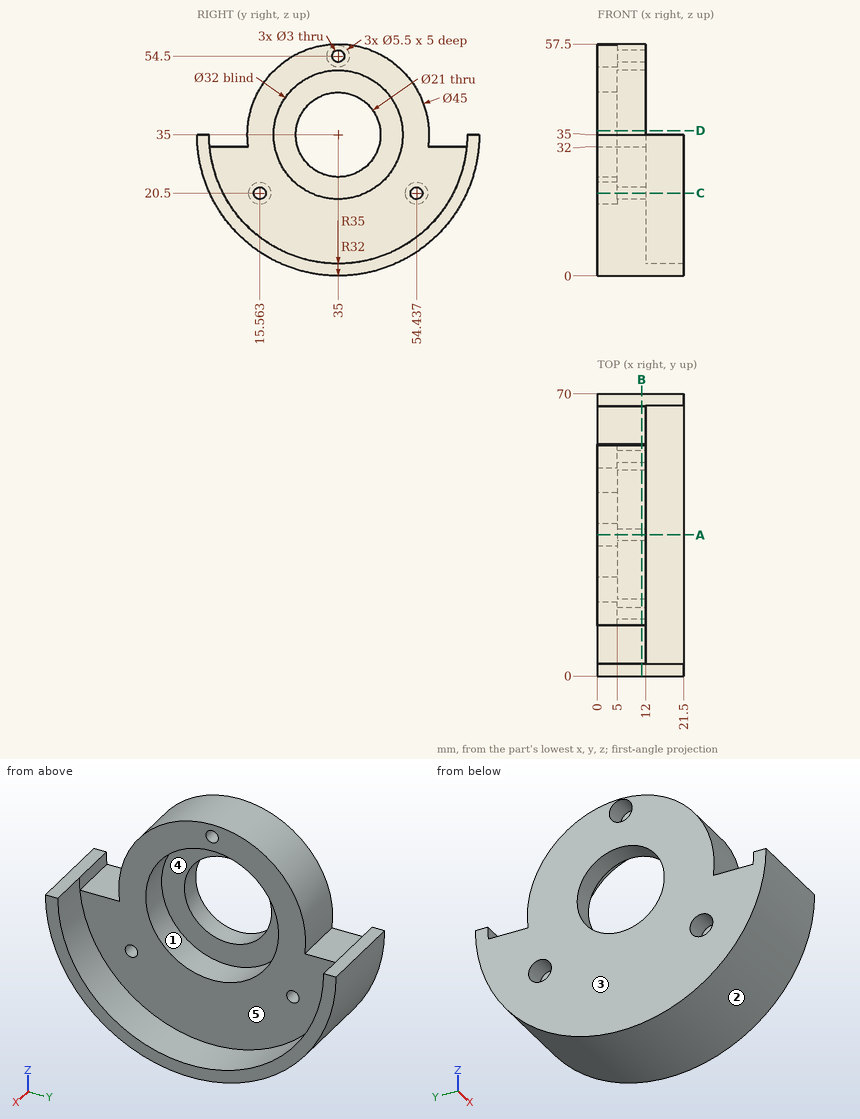
Geometry: see drawing. Coordinates: mm, zero at the bounding-box minimum. A direction names the side the tool comes from. Give positions to 0.01 mm unless a question says otherwise; leave off trailing zeros. Loops run counter-clockwise (first coordinate to the right, second up) from the corner with the lowest first, then second, coordinate; pieces in that order, holes last. Notation, with made-up numbers: (78, 14) - (101, 14) arc R14 cw to (101, 40) - close; hole circle Ø5 at (85, -30.75). An arc over 180 degrees is marked (long way). Use CSV: the item, a comma, the result in double quotes. Start each with the question number.
Item 1: Section C-C on z = 20.5. Return loops of the section in (x, y) (1 decimal).
Item 2: Section D-D on z = 36. Return loops of the section in (x, y).
Item 3: Mould query, pull axis Z, two halves, no side actions, for the marked faces 1, 2 and 3. Classes: pulls with the +Z half, pulls with the -Z half, needs draft (parallel to the pull), parting line crosses it, or undercut.
Item 4: Contact query for flat-ended pins moving along their axis: P1, Ø3, axis at y = 32, z = 41.5, coming from the -X side; P2, Ø10.5, axis at x = 5, y = 63.5, coming from the +Z side; P3, Ø8, axis at x = 12.5, z = 8, coming from the -Y side; P4, Ø4, axis at x = 11.5, z = 24, coming from the -Y side. Output: stop coordinate, or through.
Item 5: Section B-B on x = 11. Return loops of the section in (y, z).
Item 6: Line query: line 1 (Z direction, x = 8.75, y = 34.5) (1 decimal); line 2 (Y direction, x = 7.25, z = 20.5) (1 decimal); line 3 (X direction, y = 49, z = 15). Output: solid intervals per line, ascending.
Item 7: Reachability of the marked faces 4 and 5 from +Z, -Z, +X, -X, +Y, -Y: full face, straight path, thin tool, end or side. Return the list, or none.
Item 8: Section A-A on y = 35. Return loops of the section in (x, z).
Ans:
1,outline,"(0, 3.1) - (21.5, 3.1) - (21.5, 6.5) - (12, 6.5) - (12, 14.1) - (5, 14.1) - (5, 12.8) - (0, 12.8) - close; (0, 18.3) - (5, 18.3) - (5, 17.1) - (12, 17.1) - (12, 28.2) - (5, 28.2) - (5, 41.8) - (12, 41.8) - (12, 52.9) - (5, 52.9) - (5, 51.7) - (0, 51.7) - close; (0, 57.2) - (5, 57.2) - (5, 55.9) - (12, 55.9) - (12, 63.5) - (21.5, 63.5) - (21.5, 66.9) - (0, 66.9) - close"
2,outline,"(0, 12.52) - (12, 12.52) - (12, 19.03) - (5, 19.03) - (5, 24.55) - (0, 24.55) - close; (0, 45.45) - (5, 45.45) - (5, 50.97) - (12, 50.97) - (12, 57.48) - (0, 57.48) - close"
3,face 1,"undercut"
3,face 2,"pulls with the -Z half"
3,face 3,"needs draft"
4,P1,"passes through"
4,P2,"stops at z = 35"
4,P3,"stops at y = 8.62"
4,P4,"stops at y = 1.18"
5,outline,"(0, 35) arc R35 ccw to (70, 35) - (67, 35) arc R32 cw to (66.86, 32) - (57.3, 32) arc R22.5 ccw (long way) to (12.7, 32) - (3.14, 32) arc R32 cw to (3, 35) - close; hole circle Ø3 at (15.56, 20.5); hole circle Ø32 at (35, 35); hole circle Ø3 at (35, 54.5); hole circle Ø3 at (54.44, 20.5)"
6,line 1,"z = 0 to 19, 51 to 53.1, 55.9 to 57.5"
6,line 2,"y = 3.1 to 14.1, 17.1 to 28.2, 41.8 to 52.9, 55.9 to 66.9"
6,line 3,"x = 0 to 12"
7,face 4,"+X"
7,face 5,"+Z, +X"
8,outline,"(0, 0) - (21.5, 0) - (21.5, 3) - (12, 3) - (12, 19) - (5, 19) - (5, 24.5) - (0, 24.5) - close; (0, 45.5) - (5, 45.5) - (5, 51) - (12, 51) - (12, 53) - (5, 53) - (5, 51.75) - (0, 51.75) - close; (0, 57.25) - (5, 57.25) - (5, 56) - (12, 56) - (12, 57.5) - (0, 57.5) - close"
